The model under review builds one solid part; all positions refer to its coordinate system, in mm. A direction names the side the tool comes from. Round coordinates to 2 decimals unless told otherwise and drop trailing zeros. Order: outer loops, then holes, each group sorted by start corner. A loop starts at its lowest first (then second) coordinate and runs counter-clockwise, first axis right, second up. Notation, with made-up numbers: (48, 15.25) -> (87, 15.25) arc R31 ccw to (87, 53.25) -> close; hole circle Ø11 at (12, 42.5). An arc over 180 degrees is marked (long way). Use a Markdown table: item, result. Add a question column.
```python
from build123d import *

# Parameters (mm, degrees)
F0_W     = 48.751022
F0_H     = 51.794138
F1_DEPTH = 25
F2_W     = 31.759218
F2_H     = 31.388528
F3_DEPTH = 4
F4_R     = 11.712322
F5_DEPTH = 650


with BuildPart() as f1:
    # F0 (on Top) → F1 (new body)
    with BuildSketch(Plane.XY):
        Rectangle(F0_W, F0_H)
    extrude(amount=F1_DEPTH)

    # F2 (on face) → F3 (join)
    with BuildSketch(Plane(origin=(0, 0, 0), x_dir=(1, 0, 0), z_dir=(0, 0, -1))):
        Rectangle(F2_W, F2_H)
    extrude(amount=F3_DEPTH)

    # F4 (on face) → F5 (join)
    with BuildSketch(Plane(origin=(0, 0, -4), x_dir=(1, 0, 0), z_dir=(0, 0, -1))):
        Circle(F4_R)
    extrude(amount=F5_DEPTH)


solid = f1.part
```
Q1. Wall thickness on line 1 (Z direction, x = 13.5, y = 2.5); line 2 (Y direction, x = -0.5, z = -236.5); line 3 (Z direction, x = 14, y = -22): over which ranges is each line inside the solid? List them lowest first. Write a range as [from, to].
Q2. Insertion check: pin 1 (3 mm diameter, centred on x = 1.5, z = -2, fed in from -Y); pin 2 (5 mm diameter, centred on x = 8.5, z = -550.5, fed in from +Y); pin 3 (1 mm diameter, centred on y = -10.5, z = -527.5, fed in from -X). Each pin has a flat end and moves straight along its axis. Give the tip position at first contact, or say it passes through.
Q3. Machinability: for faces 1 (the flat face through (7, -11, -4)), 2 (the flat face through (24.376, 0, 12)), which of the approach directions +Z, -Z, +X, -X, +Y, -Y give a long, thin tool a straight path to every point of the face, cutting with its end or side? Answer none if there is none.
Q4. Add section B-B (y = 0). Write out the cut boundary in (x, z).
Q5. Add section C-C (z = -257). Write out the cut boundary in (x, y), then the cut area to 3 significant figures.
Q6. Add section A-A (x = 0). Write out the cut boundary in (y, z), then the cut area to 3 significant figures.
Report:
| question | item | result |
|---|---|---|
| 1 | line 1 | z = [-4, 25] |
| 1 | line 2 | y = [-11.7, 11.7] |
| 1 | line 3 | z = [0, 25] |
| 2 | pin 1 | stops at y = -15.69 |
| 2 | pin 2 | stops at y = 10.06 |
| 2 | pin 3 | stops at x = -6.1 |
| 3 | face 1 | -Z |
| 3 | face 2 | +Z, -Z, +X, +Y, -Y |
| 4 | outline | (-24.38, 0) -> (-15.88, 0) -> (-15.88, -4) -> (-11.71, -4) -> (-11.71, -654) -> (11.71, -654) -> (11.71, -4) -> (15.88, -4) -> (15.88, 0) -> (24.38, 0) -> (24.38, 25) -> (-24.38, 25) -> close |
| 5 | outline | circle Ø23.42 at (0, 0) |
| 5 | area | 431 mm² |
| 6 | outline | (-25.9, 0) -> (-15.69, 0) -> (-15.69, -4) -> (-11.71, -4) -> (-11.71, -654) -> (11.71, -654) -> (11.71, -4) -> (15.69, -4) -> (15.69, 0) -> (25.9, 0) -> (25.9, 25) -> (-25.9, 25) -> close |
| 6 | area | 16,600 mm² |
